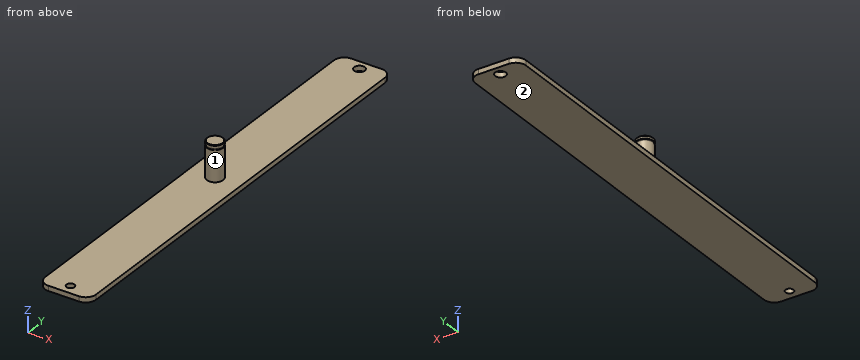
from build123d import *

# Parameters (mm, degrees)
F0_W     = 50
F0_H     = 5
F1_DEPTH = 440
F2_R     = 5.25
F2_R_2   = 3.9261217041
F3_DEPTH = 5.001
F4_R     = 8
F5_DEPTH = 35
F6_R     = 10
F8_R     = 8
F8_R_2   = 7.5
F9_DEPTH = 1.5
F10_SIZE = 0.5


with BuildPart() as f1:
    # F0 (on Front) → F1 (new body)
    with BuildSketch(Plane.XZ):
        Rectangle(F0_W, F0_H)
    extrude(amount=F1_DEPTH)

    # F2 (on face) → F3 (cut, through all)
    with BuildSketch(Plane.XY.offset(2.5)):
        with Locations((0, -10)):
            Circle(F2_R)
        with Locations((0, -430)):
            Circle(F2_R_2)
    extrude(amount=-F3_DEPTH, mode=Mode.SUBTRACT)

    # F4 (on face) → F5 (join)
    with BuildSketch(Plane.XY.offset(2.5)):
        with Locations((0, -220)):
            Circle(F4_R)
    extrude(amount=F5_DEPTH)

    # F6
    f6_edges = [f1.edges().sort_by_distance(p)[0] for p in [
        (-25, -440, 0),
        (25, -440, 0),
        (25, 0, 0),
        (-25, 0, 0),
    ]]
    fillet(f6_edges, radius=F6_R)

    # F8 (on offset) → F9 (cut)
    with BuildSketch(Plane.XY.offset(34.5)):
        with Locations((0, -220)):
            Circle(F8_R)
        with Locations((0, -220)):
            Circle(F8_R_2, mode=Mode.SUBTRACT)
    extrude(amount=-F9_DEPTH, mode=Mode.SUBTRACT)

    # F10
    f10_edges = [f1.edges().sort_by_distance(p)[0] for p in [
        (-8, -220, 37.5),
    ]]
    chamfer(f10_edges, length=F10_SIZE)


solid = f1.part
Source: CAD feature listing. Evaluate the final solid. Frame: model axes, mm. Face numbers are marked on the shaded views. A direction names the side the tool comes from. Give positions to 0.01 mm unless a question says otherwise; leave off trailing zeros. Write each loop counter-clockwise with the first axis right and the second up, starting at its lowest first coordinate (ties: lowest second). Pieces come first, ordered by that corner, then holes. Notation, with made-up numbers: M 74,73.25 L 122,73.25 A34 ccw 122,107.25 Z; hole C 76.5,-7.5 d10. An arc over 180 degrees is marked long. Return JSON: item names as keys, results as strings. Group by question number.
1) Set-up query: the marked faces 1 and 2. Return all of +Z, -Z, +X, -X, +Y, -Y with unobstructed straight access to the full face (end or side cutting, diameter ignored); none if empty.
2) Cut plane C-C, the plane z = 11. Output: boundary loops of the cut face in (x, y), plus the area to 3 significant figures.
3) Material intervals for line 1 along Y through (x, z) = (0, 0.35); line 2 along X through (y, z) = (-430, 0.2); line 3 along Z through (x, y) = (12.5, -358.5), sorted ascending. Write a range as [from, to].
4) Pin query (flat end, axial travel): P1, Ø2, axis at x = -5.5, z = 30, coming from the +Y side; P2, Ø10, axis at x = 3.5, y = -317, coming from the +Z side; P3, Ø5, axis at y = -109.5, z = 4.5, coming from the +X side. Return the tip coordinate at first contact, or that it passes through.
5) Cut plane B-B, the plane y = -220. Output: boundary loops of the cut face in (x, z).
6) Cut plane A-A, the plane x = 0. Output: boundary loops of the cut face in (y, z), plus the area to 3 significant figures.
Recorded:
{
 "1": {"face 1": "+Z", "face 2": "-Z, +X, -X, +Y, -Y"},
 "2": {"outline": "C 0,-220 d16", "area": "201 mm²"},
 "3": {"line 1": "y = [-440, -433.93], [-426.07, -15.25], [-4.75, 0]", "line 2": "x = [-25, -3.93], [3.93, 25]", "line 3": "z = [-2.5, 2.5]"},
 "4": {"P1": "stops at y = -213.39", "P2": "stops at z = 2.5", "P3": "stops at x = 25"},
 "5": {"outline": "M -25,-2.5 L 25,-2.5 L 25,2.5 L 8,2.5 L 8,33 L 7.5,33 L 7.5,34.5 L 8,34.5 L 8,37 L 7.5,37.5 L -7.5,37.5 L -8,37 L -8,34.5 L -7.5,34.5 L -7.5,33 L -8,33 L -8,2.5 L -25,2.5 Z"},
 "6": {"outline": "M -440,-2.5 L -433.93,-2.5 L -433.93,2.5 L -440,2.5 Z; M -426.07,-2.5 L -15.25,-2.5 L -15.25,2.5 L -212,2.5 L -212,33 L -212.5,33 L -212.5,34.5 L -212,34.5 L -212,37 L -212.5,37.5 L -227.5,37.5 L -228,37 L -228,34.5 L -227.5,34.5 L -227.5,33 L -228,33 L -228,2.5 L -426.07,2.5 Z; M -4.75,-2.5 L 0,-2.5 L 0,2.5 L -4.75,2.5 Z", "area": "2,670 mm²"}
}
